Verification items for this drawing (mm, ordinates from the low corner). A direction names the side the tool comes from. Round coordinates to 2 decimals unless told otherwise and drop trailing zeros. Order: outer loops, then holes, each group sorted by start corner. A loop starts at its lowest first (then second) coordinate and runs counter-clockwise, first axis right, second up. Notation, with made-up numbers: M 61.25,3 L 107.25,3 A21 cw 107.25,42 Z; hole C -31.75,73 d2. An arc over 180 degrees is marked long. Return JSON: item names as keys, results as strings. Group by question number.
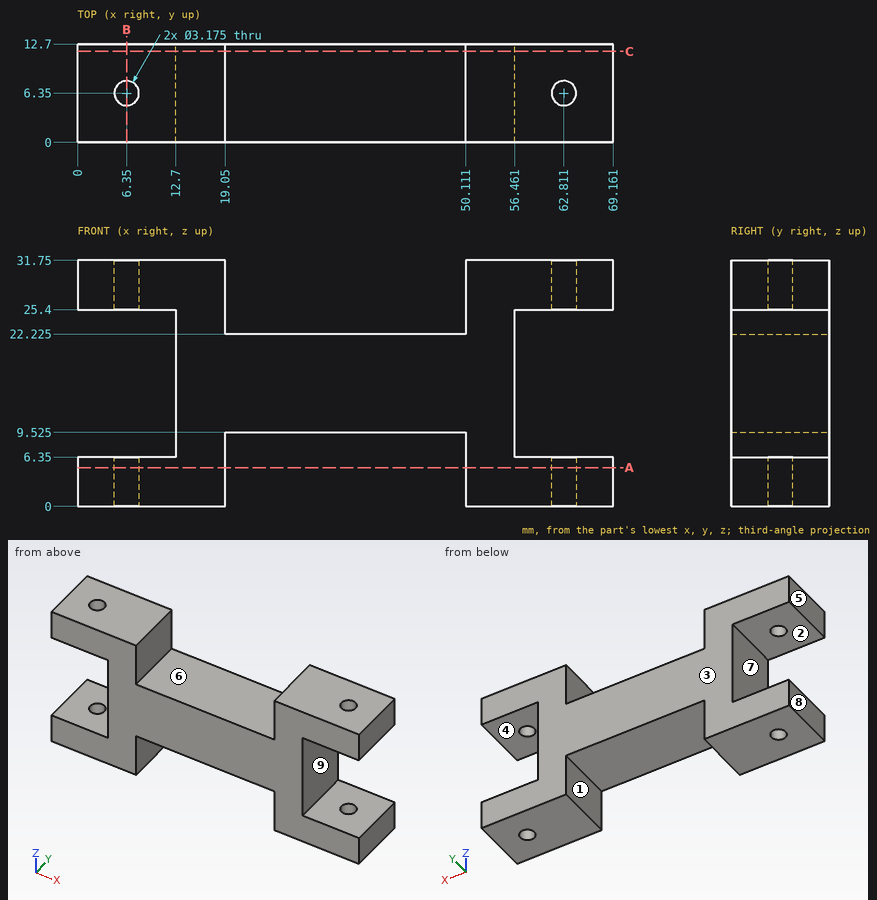
1. Cross-section at B-B (x = 6.35). Enter the section's corners in (y, z).
2. Access from +Z, -Z, +X, -X, +Y, -Y to the whole of each face (thin tool, end or side, straight path). Record for the marked faces 1, 2, 3, 4 and 5.
3. Cross-section at A-A (z = 5). Give the number of separate pieces and of enclosed holes in the cut face, plus the area to 3 significant figures.
4. Thickness scan on line 1 along Z through (x, y) = (56.5, 6.5); line 2 along X through (y, z) = (4.25, 2.5); line 3 along X through (y, z) = (0.5, 24). Record the ranges inside material, lowest first. Write a range as from..to.
5. Draft check along Z on the marked faces 6, 7, 8 and 9. Enter one of: +Z half, -Z half, draft (parallel to the pull), parting line (faces both ways), or undercut.
6. Cross-section at C-C (y = 11.75). Enter the section's corners in (x, z) (3 decimals).
7. Go/stop test with flat-tipped pins: pin 1 (2.5 mm diameter, centred on x = 62.81, y = 6.35, fed in from +Z); pin 2 (3 mm diameter, centred on x = 44.5, y = 3.5, fed in from +Z) (3 decimals); pin 3 (6.5 mm diameter, centred on x = 6.5, y = 5, fed in from +Z); pin 4 (6.5 mm diameter, centred on y = 4.5, z = 20, fed in from -X). Record where each tip stops, or that it passes through.
Computed:
{
 "1": {"outline": "M 0,0 L 4.76,0 L 4.76,6.35 L 0,6.35 Z; M 0,25.4 L 4.76,25.4 L 4.76,31.75 L 0,31.75 Z; M 7.94,0 L 12.7,0 L 12.7,6.35 L 7.94,6.35 Z; M 7.94,25.4 L 12.7,25.4 L 12.7,31.75 L 7.94,31.75 Z"},
 "2": {"face 1": "-Z, +Y, -Y", "face 2": "-X, +Y, -Y", "face 3": "+Z, -Z, +X, -X, +Y", "face 4": "+X, +Y, -Y", "face 5": "+Z, -Z, -X, +Y, -Y"},
 "3": {"separate pieces": "2", "enclosed holes": "2", "area": "468 mm²"},
 "4": {"line 1": "z = 0..6.35, 25.4..31.75", "line 2": "x = 0..19.05, 50.11..69.16", "line 3": "x = 12.7..19.05, 50.11..56.46"},
 "5": {"face 6": "+Z half", "face 7": "undercut", "face 8": "draft", "face 9": "undercut"},
 "6": {"outline": "M 0,0 L 19.05,0 L 19.05,9.525 L 50.111,9.525 L 50.111,0 L 69.161,0 L 69.161,6.35 L 56.461,6.35 L 56.461,25.4 L 69.161,25.4 L 69.161,31.75 L 50.111,31.75 L 50.111,22.225 L 19.05,22.225 L 19.05,31.75 L 0,31.75 L 0,25.4 L 12.7,25.4 L 12.7,6.35 L 0,6.35 Z"},
 "7": {"pin 1": "passes through", "pin 2": "stops at z = 22.225", "pin 3": "stops at z = 31.75", "pin 4": "stops at x = 12.7"}
}
